For this review, take the finished solid that the model builds, in its own axes (mm). A direction names the side the tool comes from. Coordinates: 2 decimals unless noted, no trailing zeros. Loops run counter-clockwise (first coordinate to the right, second up) from the corner with the lowest first, then second, coordinate; pieces in that order, holes last. Notation, with made-up numbers: (81.5, -16.75) - (106.5, -16.75) arc R26 ccw to (106.5, 11.25) - close; hole circle Ø2 at (86, 49.25). An arc over 180 degrees is marked (long way). Answer as a JSON object with one key per item and string values. Group by question number.
Item 1: We need section A-A (x = -7.5). Give the boundary of the cut face in (y, z), then the cut area to 3 significant figures.
Item 2: To check wall thickness, follow line 1 (X direction, y = 4.76, z = -36); line 2 (Y direction, x = -15, z = -38); line 3 (Z direction, x = 3.75, y = 4.76). State the ranges of each line that lie inside material, in increasing order.
Item 3: Tool access review of faces 5 (the cylindrical face through (17.48, 4.43, -37.1)), 6 (the flat face through (-43, 5, -1.96)), 7 (the flat face through (21.511, 5, 0)), 8 (the flat face through (42, 5, -1.96)): name each direction out of +Z, -Z, +X, -X, +Y, -Y from which nothing blocks a thin tool from reaching the whole face with its end or side.
Item 4: We need section D-D (y = 4.76). State how many separate pieces and enclosed holes the cut face has, then the cut area to 3 significant figures.
Item 5: We need section C-C (x = 15). Give the boundary of the cut face in (y, z), then the cut area to 3 significant figures.
Item 6: Clearance check with flat-ended pins moving along their axes: pin 1 (2.5 mm diameter, centred on x = -46, y = 5, fed in from -Z); pin 2 (1 mm diameter, centred on y = 7.5, z = 12.5, fed in from -X); pin 3 (4.5 mm diameter, centred on x = 15, y = 4.76, fed in from +Z). State where each tip first meets the part, or that it passes through.
Item 7: We need section B-B (z = -3.5). Give the boundary of the cut face in (x, y).
Item 8: Mouldability with a two-part tool opening along Z and no side actions: class faces 1 (the flat face through (-45, 5, -26.96)), 2 (the cylindrical face through (-42.52, 4.43, -37.1)), 3 (the flat face through (-6, 5, 38.572)), 4 (the cylindrical face through (20.008, 4.693, 20.147)) as released by +Z, released by -Z, zero draft, split by the parting line, or undercut.
from build123d import *

# Parameters (mm, degrees)
ESBO_O1_W                    = 60
ESBO_O1_H                    = 50
RESSALTO_EXTRUS_O1_DEPTH     = 9.52
CORTE_EXTRUS_O1_DEPTH        = 9.52
CORTE_EXTRUS_O1_START        = 7.26
CORTE_EXTRUS_O1_2_DEPTH      = 2.26
CORTE_EXTRUS_O1_3_DEPTH      = 2.2599999
CORTE_EXTRUS_O1_START_2      = -30
CORTE_EXTRUS_O1_4_OUTLINE_W  = 5.0000001
CORTE_EXTRUS_O1_4_OUTLINE_H  = 3.572491942
CORTE_EXTRUS_O1_4_DEPTH      = 28
CORTE_EXTRUS_O1_START_3      = 2
CORTE_EXTRUS_O1_5_OUTLINE_W  = 5.0000001
CORTE_EXTRUS_O1_5_OUTLINE_H  = 3.572491942
CORTE_EXTRUS_O1_5_DEPTH      = 28
CORTE_EXTRUS_O1_START_4      = -10
CORTE_EXTRUS_O1_6_DEPTH      = 8
CORTE_EXTRUS_O1_7_DEPTH      = 8
CORTE_EXTRUS_O1_START_5      = -46.96
CORTE_EXTRUS_O1_8_DEPTH      = 21.96
CORTE_EXTRUS_O1_START_6      = -26.96
CORTE_EXTRUS_O1_9_OUTLINE_W  = 25
CORTE_EXTRUS_O1_9_OUTLINE_H  = 5.0000001
CORTE_EXTRUS_O1_9_DEPTH      = 25
CORTE_EXTRUS_O1_10_OUTLINE_R = 2.5
CORTE_EXTRUS_O1_10_DEPTH     = 1.96


with BuildPart() as part:
    # Esboço1 → Ressalto-extrusão1 (new body)
    with BuildSketch(Plane(origin=(0, 0, 0), x_dir=(1, 0, 0), z_dir=(0, 1, 0))):
        Rectangle(ESBO_O1_W, ESBO_O1_H)
    extrude(amount=RESSALTO_EXTRUS_O1_DEPTH)

    # Corte-extrusão1: read off the stored shape, not the designer's step
    # Corte-extrusão1 outline → Corte-extrusão1 (cut)
    with BuildSketch(Plane(origin=(0, 0, 0), x_dir=(1, 0, 0), z_dir=(0, 1, 0))):
        with BuildLine():
            ThreePointArc((-16.551848481, -21.569831255), (-16.522584074, -21.571242343), (-16.493312326, -21.572491942))
            Line((-16.493312326, -21.572491942), (-2, -21.572491942))
            Line((-2, -21.572491942), (-2, -25))
            Line((-2, -25), (2, -25))
            Line((2, -25), (2, -21.572491942))
            Line((2, -21.572491942), (16.511245971, -21.572491942))
            ThreePointArc((16.511245971, -21.572491942), (20.046779877, -20.108025848), (21.511245971, -16.572491942))
            Line((21.511245971, -16.572491942), (21.511245971, 16.45))
            ThreePointArc((21.511245971, 16.45), (20.037938418, 20.019740143), (16.469538401, 21.496290566))
            Line((16.469538401, 21.496290566), (-16.430461599, 21.496290566))
            ThreePointArc((-16.430461599, 21.496290566), (-20.093320705, 20.064258273), (-21.587468917, 16.426295322))
            Line((-21.587468917, 16.426295322), (-21.587468917, -16.473704678))
            ThreePointArc((-21.587468917, -16.473704678), (-20.959260779, -18.779602466), (-19.383464148, -20.576453893))
            ThreePointArc((-19.383464148, -20.576453893), (-18.043937425, -21.290581379), (-16.551848481, -21.569831255))
        make_face()
    extrude(amount=CORTE_EXTRUS_O1_DEPTH, mode=Mode.SUBTRACT)

    # Corte-extrus_o1 2 outline → Corte-extrus_o1 2 (add)
    with BuildSketch(Plane(origin=(0, 0, 0), x_dir=(1, 0, 0), z_dir=(0, 1, 0)).offset(CORTE_EXTRUS_O1_START)):
        Polygon((-2, -38.572491942), (-2, -25), (-30, -25), (-30, -28.572491942), (-10, -28.572491942), (-10, -38.572491942), align=None)
        Polygon((30, -25), (2, -25), (2, -38.572491942), (10, -38.572491942), (10, -28.572491942), (30, -28.572491942), align=None)
        Polygon((-55, 1.96), (-30, 1.96), (-30, 25), (30, 25), (30, 1.96), (55, 1.96), (55, 46.96), (-55, 46.96), align=None)
    extrude(amount=CORTE_EXTRUS_O1_2_DEPTH)

    # Corte-extrus_o1 3 outline → Corte-extrus_o1 3 (add)
    with BuildSketch(Plane(origin=(0, 0, 0), x_dir=(1, 0, 0), z_dir=(0, 1, 0))):
        Polygon((-2, -38.572491942), (-2, -25), (-30, -25), (-30, -28.572491942), (-10, -28.572491942), (-10, -38.572491942), align=None)
        Polygon((30, -25), (2, -25), (2, -38.572491942), (10, -38.572491942), (10, -28.572491942), (30, -28.572491942), align=None)
        Polygon((-55, 1.96), (-30, 1.96), (-30, 25), (30, 25), (30, 1.96), (55, 1.96), (55, 46.96), (-55, 46.96), align=None)
    extrude(amount=CORTE_EXTRUS_O1_3_DEPTH)

    # Corte-extrus_o1 4 outline → Corte-extrus_o1 4 (add)
    with BuildSketch(Plane.YZ.offset(CORTE_EXTRUS_O1_START_2)):
        with Locations((4.75999995, 26.786245971)):
            Rectangle(CORTE_EXTRUS_O1_4_OUTLINE_W, CORTE_EXTRUS_O1_4_OUTLINE_H)
    extrude(amount=CORTE_EXTRUS_O1_4_DEPTH)

    # Corte-extrus_o1 5 outline → Corte-extrus_o1 5 (add)
    with BuildSketch(Plane.YZ.offset(CORTE_EXTRUS_O1_START_3)):
        with Locations((4.75999995, 26.786245971)):
            Rectangle(CORTE_EXTRUS_O1_5_OUTLINE_W, CORTE_EXTRUS_O1_5_OUTLINE_H)
    extrude(amount=CORTE_EXTRUS_O1_5_DEPTH)

    # Corte-extrus_o1 6 outline → Corte-extrus_o1 6 (add)
    with BuildSketch(Plane.YZ.offset(CORTE_EXTRUS_O1_START_4)):
        with BuildLine():
            Line((7.26, 28.572491942), (7.26, 33.572491942))
            ThreePointArc((7.26, 33.572491942), (4.76, 31.072491942), (2.26, 33.572491942))
            Line((2.26, 33.572491942), (2.2599999, 28.572491942))
            Line((2.2599999, 28.572491942), (7.26, 28.572491942))
        make_face()
        with BuildLine():
            ThreePointArc((2.26, 33.572491942), (4.76, 36.072491942), (7.26, 33.572491942))
            Line((7.26, 33.572491942), (7.26, 38.572491942))
            Line((7.26, 38.572491942), (2.2599999, 38.572491942))
            Line((2.2599999, 38.572491942), (2.26, 33.572491942))
        make_face()
    extrude(amount=CORTE_EXTRUS_O1_6_DEPTH)

    # Corte-extrus_o1 7 outline → Corte-extrus_o1 7 (add)
    with BuildSketch(Plane.YZ.offset(CORTE_EXTRUS_O1_START_3)):
        with BuildLine():
            Line((7.26, 28.572491942), (7.26, 33.572491942))
            ThreePointArc((7.26, 33.572491942), (4.76, 31.072491942), (2.26, 33.572491942))
            Line((2.26, 33.572491942), (2.2599999, 28.572491942))
            Line((2.2599999, 28.572491942), (7.26, 28.572491942))
        make_face()
        with BuildLine():
            ThreePointArc((2.26, 33.572491942), (4.76, 36.072491942), (7.26, 33.572491942))
            Line((7.26, 33.572491942), (7.26, 38.572491942))
            Line((7.26, 38.572491942), (2.2599999, 38.572491942))
            Line((2.2599999, 38.572491942), (2.26, 33.572491942))
        make_face()
    extrude(amount=CORTE_EXTRUS_O1_7_DEPTH)

    # Corte-extrus_o1 8 outline → Corte-extrus_o1 8 (add)
    with BuildSketch(Plane.XY.offset(CORTE_EXTRUS_O1_START_5)):
        with BuildLine():
            ThreePointArc((45, 7.26), (47.5, 4.76), (45, 2.26))
            Line((45, 2.26), (55, 2.2599999))
            Line((55, 2.2599999), (55, 7.26))
            Line((55, 7.26), (45, 7.26))
        make_face()
        with BuildLine():
            ThreePointArc((45, 2.26), (42.5, 4.76), (45, 7.26))
            Line((45, 7.26), (15.000000025, 7.26))
            ThreePointArc((15.000000025, 7.26), (17.5, 4.759999988), (15.000000001, 2.26))
            Line((15.000000001, 2.26), (45, 2.26))
        make_face()
        with BuildLine():
            ThreePointArc((15.000000001, 2.26), (12.5, 4.760000012), (15.000000025, 7.26))
            Line((15.000000025, 7.26), (-15.000000034, 7.26))
            ThreePointArc((-15.000000034, 7.26), (-12.5, 4.760000017), (-15, 2.26))
            Line((-15, 2.26), (15.000000001, 2.26))
        make_face()
        with BuildLine():
            ThreePointArc((-15, 2.26), (-17.5, 4.759999983), (-15.000000034, 7.26))
            Line((-15.000000034, 7.26), (-44.999999984, 7.26))
            ThreePointArc((-44.999999984, 7.26), (-42.5, 4.759999992), (-45, 2.26))
            Line((-45, 2.26), (-15, 2.26))
        make_face()
        with BuildLine():
            ThreePointArc((-45, 2.26), (-47.5, 4.760000008), (-44.999999984, 7.26))
            Line((-44.999999984, 7.26), (-55, 7.26))
            Line((-55, 7.26), (-55, 2.2599999))
            Line((-55, 2.2599999), (-45, 2.26))
        make_face()
    extrude(amount=CORTE_EXTRUS_O1_8_DEPTH)

    # Corte-extrus_o1 9 outline → Corte-extrus_o1 9 (add)
    with BuildSketch(Plane.XY.offset(CORTE_EXTRUS_O1_START_6)):
        with Locations((42.5, 4.75999995)):
            Rectangle(CORTE_EXTRUS_O1_9_OUTLINE_W, CORTE_EXTRUS_O1_9_OUTLINE_H)
        with Locations((-42.5, 4.75999995)):
            Rectangle(CORTE_EXTRUS_O1_9_OUTLINE_W, CORTE_EXTRUS_O1_9_OUTLINE_H)
    extrude(amount=CORTE_EXTRUS_O1_9_DEPTH)

    # Corte-extrus_o1 10 outline → Corte-extrus_o1 10 (add)
    with BuildSketch(Plane.XY.offset(CORTE_EXTRUS_O1_START_6)):
        with Locations((15, 4.76)):
            Circle(CORTE_EXTRUS_O1_10_OUTLINE_R)
        with Locations((-15, 4.76)):
            Circle(CORTE_EXTRUS_O1_10_OUTLINE_R)
    extrude(amount=CORTE_EXTRUS_O1_10_DEPTH)


solid = part.part
Check sheet entries:
{
 "1": {"outline": "(0, -46.96) - (9.52, -46.96) - (9.52, -21.5) - (0, -21.5) - close; (0, 21.57) - (9.52, 21.57) - (9.52, 38.57) - (0, 38.57) - close; hole circle Ø5 at (4.76, 33.57)", "area": "385 mm2"},
 "2": {"line 1": "x = -55 to -47.5, -42.5 to -17.5, -12.5 to 12.5, 17.5 to 42.5, 47.5 to 55", "line 2": "y = 0 to 2.26, 7.26 to 9.52", "line 3": "z = -46.96 to -21.5, 21.57 to 31.07, 36.07 to 38.57"},
 "3": {"face 5": "-Z", "face 6": "+Z, -X, +Y, -Y", "face 7": "+Y, -Y", "face 8": "+Z, +X, +Y, -Y"},
 "4": {"separate pieces": "3", "enclosed holes": "0", "area": "4,600 mm2"},
 "5": {"outline": "(0, -46.96) - (2.26, -46.96) - (2.26, -26.96) - (7.26, -26.96) - (7.26, -46.96) - (9.52, -46.96) - (9.52, -21.5) - (0, -21.5) - close; (0, 21.57) - (9.52, 21.57) - (9.52, 28.57) - (0, 28.57) - close", "area": "209 mm2"},
 "6": {"pin 1": "stops at z = -26.96", "pin 2": "stops at x = -30", "pin 3": "stops at z = 28.57"},
 "7": {"outline": "(-55, 0) - (-21.59, 0) - (-21.59, 9.52) - (-55, 9.52) - close; (21.51, 0) - (55, 0) - (55, 9.52) - (21.51, 9.52) - close"},
 "8": {"face 1": "released by -Z", "face 2": "zero draft", "face 3": "released by +Z", "face 4": "undercut"}
}
